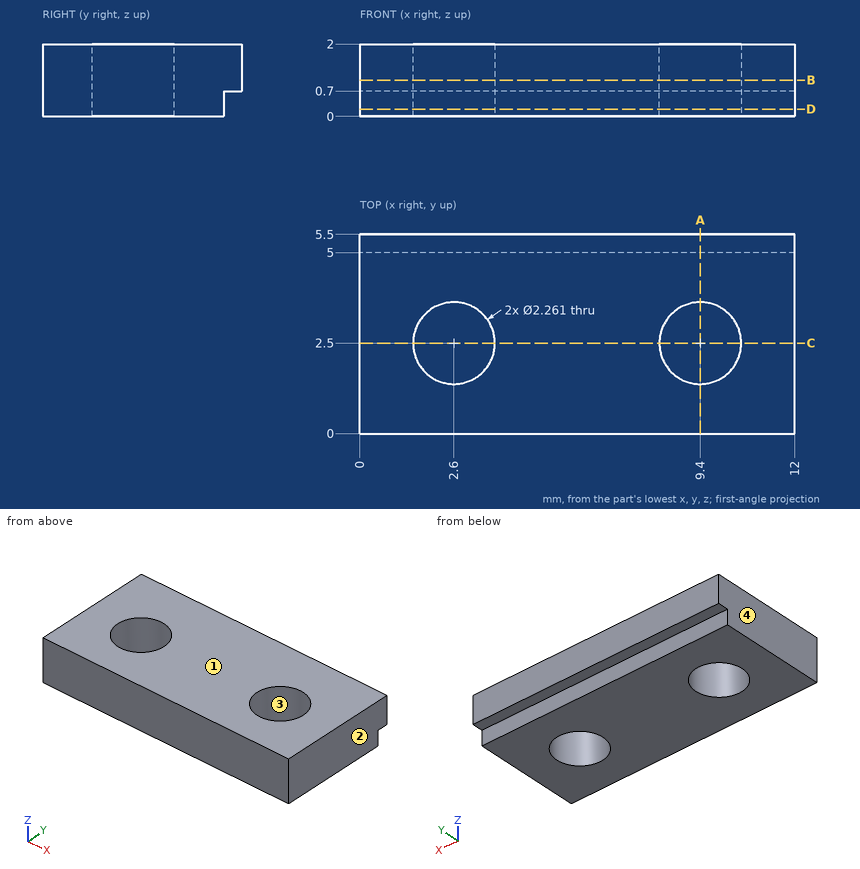
Drawing for the job (mm, zero at the part's lowest x, y, z). Coordinates: 2 decimals unless noted, no trailing zeros. Loops run counter-clockwise (first coordinate to the right, second up) from the corner with the lowest first, then second, coordinate; pieces in that order, holes last. Notation, with made-up numbers: (-29, 61) - (-24, 61) arc R17 ccw to (-24, 90) - close; hole circle Ø2 at (33, 0.5). An arc over 180 degrees is marked (long way). Return JSON: item names as keys, results as strings.
1. Mould opens along X. For the marked faces 1, 2, 3 and 4 say: released by +X, released by -X, zero draft, split by the parting line, or undercut.
Result:
{"face 1": "zero draft", "face 2": "released by +X", "face 3": "undercut", "face 4": "released by -X"}
2. Band-saw the part on A-A (x = 9.4). Give the cut face in (y, z).
Result:
{"outline": "(0, 0) - (1.37, 0) - (1.37, 2) - (0, 2) - close; (3.63, 0) - (5, 0) - (5, 0.7) - (5.5, 0.7) - (5.5, 2) - (3.63, 2) - close"}
3. Probe L1, parallel to Y at x = 2.6, z = 1.4; L2, parallel to X at y = 3.4, z = 0.85 (1 decimal); L3, parallel to Y at x = 2.6, z = 0.5. List the from-to ranges inside material, lowest first. Write a range as from..to.
Result:
{"L1": "y = 0..1.37, 3.63..5.5", "L2": "x = 0..1.9, 3.3..8.7, 10.1..12", "L3": "y = 0..1.37, 3.63..5"}
4. Band-saw the part on C-C (y = 2.5). Give the cut face in (x, z).
Result:
{"outline": "(0, 0) - (1.47, 0) - (1.47, 2) - (0, 2) - close; (3.73, 0) - (8.27, 0) - (8.27, 2) - (3.73, 2) - close; (10.53, 0) - (12, 0) - (12, 2) - (10.53, 2) - close"}
5. Band-saw the part on D-D (z = 0.2). Give the cut face in (x, y).
Result:
{"outline": "(0, 0) - (12, 0) - (12, 5) - (0, 5) - close; hole circle Ø2.26 at (2.6, 2.5); hole circle Ø2.26 at (9.4, 2.5)"}
6. Band-saw the part on B-B (z = 1). Give the cut face in (x, y).
Result:
{"outline": "(0, 0) - (12, 0) - (12, 5.5) - (0, 5.5) - close; hole circle Ø2.26 at (2.6, 2.5); hole circle Ø2.26 at (9.4, 2.5)"}
